from build123d import *

# Parameters (mm, degrees)
F0_R     = 6.35
F1_DEPTH = 4.7625


with BuildPart() as f1:
    # F0 (on Front) → F1 (new body, symmetric)
    with BuildSketch(Plane.XZ):
        with BuildLine():
            Line((-101.7769366858, -25.4), (149.4019366858, -25.4))
            ThreePointArc((149.4019366858, -25.4), (139.7, 0), (149.4019366858, 25.4))
            Line((149.4019366858, 25.4), (-101.7769366858, 25.4))
            ThreePointArc((-101.7769366858, 25.4), (-94.5830331235, 13.5949216204), (-92.075, 0))
            ThreePointArc((-92.075, 0), (-94.5830331235, -13.5949216204), (-101.7769366858, -25.4))
        make_face()
        with Locations((63.5, 0)):
            Circle(F0_R, mode=Mode.SUBTRACT)
        with BuildLine():
            Line((-130.175, -25.4), (-101.7769366858, -25.4))
            ThreePointArc((-101.7769366858, -25.4), (-94.5830331235, -13.5949216204), (-92.075, 0))
            ThreePointArc((-92.075, 0), (-94.5830331235, 13.5949216204), (-101.7769366858, 25.4))
            Line((-101.7769366858, 25.4), (-130.175, 25.4))
            ThreePointArc((-130.175, 25.4), (-112.2144877579, 17.9605122421), (-104.775, 0))
            ThreePointArc((-104.775, 0), (-112.2144877579, -17.9605122421), (-130.175, -25.4))
        make_face()
        with BuildLine():
            ThreePointArc((-130.175, 25.4), (-155.575, 0), (-130.175, -25.4))
            ThreePointArc((-130.175, -25.4), (-112.2144877579, -17.9605122421), (-104.775, 0))
            ThreePointArc((-104.775, 0), (-112.2144877579, 17.9605122421), (-130.175, 25.4))
        make_face()
        with Locations((-130.175, 0)):
            Circle(F0_R, mode=Mode.SUBTRACT)
        with BuildLine():
            Line((-130.175, 25.4), (-101.7769366858, 25.4))
            ThreePointArc((-101.7769366858, 25.4), (-130.175, 38.1), (-158.5730633142, 25.4))
            Line((-158.5730633142, 25.4), (-130.175, 25.4))
        make_face()
        with BuildLine():
            Line((-158.5730633142, -25.4), (-130.175, -25.4))
            ThreePointArc((-130.175, -25.4), (-155.575, 0), (-130.175, 25.4))
            Line((-130.175, 25.4), (-158.5730633142, 25.4))
            ThreePointArc((-158.5730633142, 25.4), (-168.275, 0), (-158.5730633142, -25.4))
        make_face()
        with BuildLine():
            ThreePointArc((-158.5730633142, -25.4), (-130.175, -38.1), (-101.7769366858, -25.4))
            Line((-101.7769366858, -25.4), (-130.175, -25.4))
            Line((-130.175, -25.4), (-158.5730633142, -25.4))
        make_face()
        with BuildLine():
            Line((203.2, 25.4), (203.2, -25.4))
            Line((203.2, -25.4), (149.4019366858, -25.4))
            ThreePointArc((149.4019366858, -25.4), (191.3949216204, -35.5919668765), (215.9, 0))
            ThreePointArc((215.9, 0), (191.3949216204, 35.5919668765), (149.4019366858, 25.4))
            Line((149.4019366858, 25.4), (203.2, 25.4))
        make_face()
        with BuildLine():
            Line((149.4019366858, -25.4), (203.2, -25.4))
            Line((203.2, -25.4), (203.2, 25.4))
            Line((203.2, 25.4), (149.4019366858, 25.4))
            ThreePointArc((149.4019366858, 25.4), (139.7, 0), (149.4019366858, -25.4))
        make_face()
        with Locations((177.8, 0)):
            Circle(F0_R, mode=Mode.SUBTRACT)
    extrude(amount=F1_DEPTH, both=True)


solid = f1.part
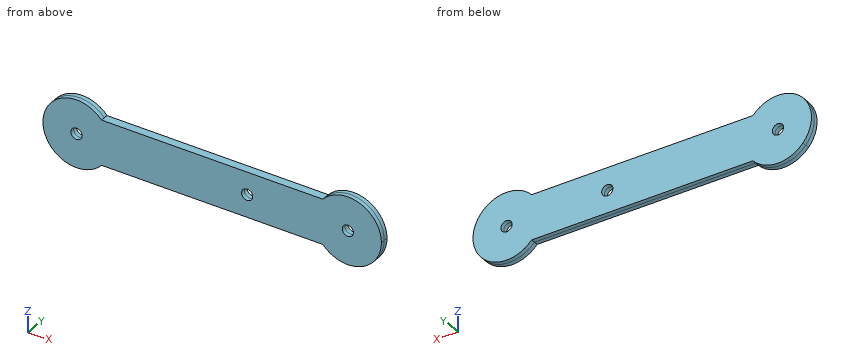
Build history of the part. All positions in model axes, mm. Round coordinates to 2 decimals unless told otherwise and drop trailing zeros. Write each loop counter-clockwise with the first axis right and the second up, starting at its lowest first coordinate (ties: lowest second). Pieces come first, ordered by that corner, then holes. Notation, with made-up numbers: (87.5, 63.25) - (116.5, 63.25) arc R11 cw to (116.5, 78.25) - close; hole circle Ø5 at (23, 3.5). An arc over 180 degrees is marked (long way). Use CSV: the item, a comma, the result in double quotes.
(1) Pin check, flat tips, straight feed: P1, Ø4, axis at y = 2.5, z = 26.5, coming from the +X side; P2, Ø16.5, axis at x = 177.8, z = 0, coming from the -Y side; P3, Ø4, axis at y = 2.5, z = -10.5, coming from the +X side; P4, Ø3, axis at x = 93.5, y = 2, coming from the -Z side. Stop position of each tip, or through.
Response:
P1,"x = 206.98"
P2,"y = -4.76"
P3,"x = 214.94"
P4,"z = -25.4"
(2) Band-saw the part on D-D (z = 21.5). Write the cut outline in (x, y), plus the area to 3 significant figures.
Response:
outline,"(-161.63, -4.76) - (209.25, -4.76) - (209.25, 4.76) - (-161.63, 4.76) - close"
area,"3,530 mm²"
(3) Wall check: line 1 (Z direction, x = 34, y = 1.75); line 2 (X direction, y = -1.25, z = 2); line 3 (X direction, y = -1, z = 35). Give the ranges that are in metal, low to high.
Response:
line 1,"-25.4 to 25.4"
line 2,"-168.22 to -136.2, -124.15 to 57.47, 69.53 to 171.77, 183.83 to 215.85"
line 3,"-145.23 to -115.12, 162.75 to 192.85"
(4) Band-saw the part on C-C (z = -30). Write the cut outline in (x, y).
Response:
outline,"(-153.66, -4.76) - (-106.69, -4.76) - (-106.69, 4.76) - (-153.66, 4.76) - close; (154.31, -4.76) - (201.29, -4.76) - (201.29, 4.76) - (154.31, 4.76) - close"
(5) Band-saw the part on B-B (x = 63.5). Write the cut outline in (y, z).
Response:
outline,"(-4.76, -25.4) - (4.76, -25.4) - (4.76, -6.35) - (-4.76, -6.35) - close; (-4.76, 6.35) - (4.76, 6.35) - (4.76, 25.4) - (-4.76, 25.4) - close"
(6) Band-saw the part on A-A (y = 3). Write the cut outline in (x, z) (3 decimals), plus the area to 3 significant figures.
Response:
outline,"(-101.777, -25.4) - (149.402, -25.4) arc R38.1 ccw (long way) to (149.402, 25.4) - (-101.777, 25.4) arc R38.1 ccw (long way) to start; hole circle Ø12.7 at (-130.175, 0); hole circle Ø12.7 at (63.5, 0); hole circle Ø12.7 at (177.8, 0)"
area,"20,800 mm²"
